Source: CAD feature listing. Evaluate the final solid. Frame: model axes, mm. Face numbers are marked on the shaded views. A direction names the side the tool comes from. Round coordinates to 2 decimals unless told otherwise and drop trailing zeros. Loops run counter-clockwise (first coordinate to the right, second up) from the corner with the lowest first, then second, coordinate; pieces in that order, holes last.
Item 1: Access query for the marked faces 1, 2 and 3. Directions: +Z, -Z, +X, -X, +Y, -Y. A direction counts if a zero-diameter tool reaches every point of the face in a straight line with its end or side. Return the directions, or none.
Item 2: Pull-direction query (Z, two-part tool) for the marked faces 4, 5 and 6; classes: released by +Z, released by -Z, zero draft, split by the parting line, or undercut.
Item 3: Section query A-A on z = 20. Return loops of the section in (x, y), then the cut area to 3 significant figures.
Item 4: Section query B-B on y = 22.5. Return loops of the section in (x, z), then the cut area to 3 significant figures.
Item 5: Section query D-D on y = 15. Return loops of the section in (x, z).
Item 6: Ray query, L1, parallel to X at y = 21.5, z = 8.5; L2, parallel to Y at x = 46.9, z = 80; L3, parallel to Y at x = 40, z = 34.4. Return the intervals inside material, ascending.
Item 7: First-contact query: P1, Ø13, axis at x = 40, y = 65, coming from the +Z side; P2, Ø8, axis at x = 9, z = 14, coming from the +Y side; P3, Ø8, axis at y = 15, z = 80, coming from the -X side; P4, Ø1, axis at x = 41, z = 59.5, coming from the -Y side. Flat tips, straight axial feed; report the tip coordinate or a pass-through.
Item 8: Section query C-C on x = 40. Return loops of the section in (y, z).
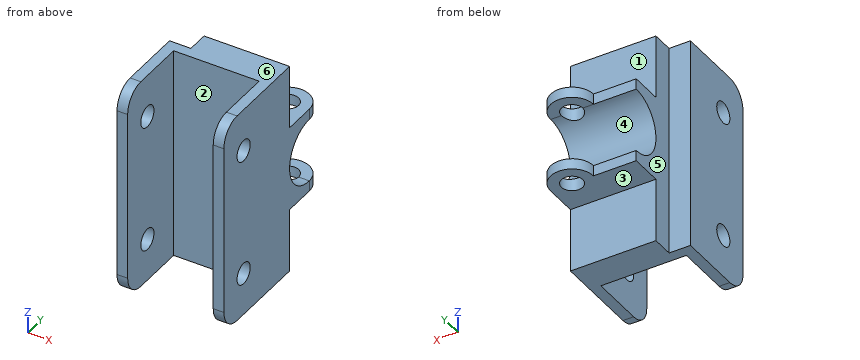
```python
from build123d import *

# Parameters (mm, degrees)
SKETCH1_R               = 5
BOSS_EXTRUDE1_DEPTH     = 100
SKETCH2_R               = 5
SKETCH2_W               = 30
SKETCH2_H               = 25
CUT_EXTRUDE1_DEPTH      = 100
FILLET1_R               = 10
SKETCH4_W               = 40
SKETCH4_H               = 100
BOSS_EXTRUDE2_DEPTH     = 10
SKETCH5_W               = 10
SKETCH5_H               = 20
CUT_EXTRUDE2_DEPTH      = 101
CUT_EXTRUDE2_DEPTH_BACK = 1
SKETCH6_W               = 10
SKETCH6_H               = 5
CUT_EXTRUDE3_DEPTH      = 1
CUT_EXTRUDE3_DEPTH_BACK = 101


with BuildPart() as part:
    # Sketch1 → Boss-Extrude1 (new body)
    with BuildSketch(Plane.XY):
        with BuildLine():
            Line((50, 0), (50, 65))
            ThreePointArc((50, 65), (40, 75), (30, 65))
            Line((30, 65), (0, 65))
            Line((0, 65), (0, 0))
            Line((0, 0), (5, 0))
            Line((5, 0), (5, 45))
            Line((5, 45), (45, 45))
            Line((45, 45), (45, 0))
            Line((45, 0), (50, 0))
        make_face()
        with Locations((40, 65)):
            Circle(SKETCH1_R, mode=Mode.SUBTRACT)
    extrude(amount=BOSS_EXTRUDE1_DEPTH)

    # Sketch2 → Cut-Extrude1 (cut)
    with BuildSketch(Plane(origin=(50, 0, 0), x_dir=(0, 0, -1), z_dir=(1, 0, 0))):
        with Locations((-80, 15)):
            Circle(SKETCH2_R)
        with Locations((-20, 15)):
            Circle(SKETCH2_R)
        with BuildLine():
            Line((-65, 65), (-65, 75))
            Line((-65, 75), (-35, 75))
            Line((-35, 75), (-35, 65))
            ThreePointArc((-35, 65), (-50, 50), (-65, 65))
        make_face()
        with Locations((-85, 62.5)):
            Rectangle(SKETCH2_W, SKETCH2_H)
        with Locations((-15, 62.5)):
            Rectangle(SKETCH2_W, SKETCH2_H)
    extrude(amount=-CUT_EXTRUDE1_DEPTH, mode=Mode.SUBTRACT)

    # Fillet1
    fillet1_edges = [part.edges().sort_by_distance(p)[0] for p in [
        (47.5, 0, 0),
        (2.5, 0, 0),
        (2.5, 0, 100),
        (47.5, 0, 100),
    ]]
    fillet(fillet1_edges, radius=FILLET1_R)

    # Sketch4 → Boss-Extrude2 (add)
    with BuildSketch(Plane.XZ.offset(-45)):
        with Locations((25, 50)):
            Rectangle(SKETCH4_W, SKETCH4_H)
    extrude(amount=BOSS_EXTRUDE2_DEPTH)

    # Sketch5 → Cut-Extrude2 (cut, two sides)
    with BuildSketch(Plane.XY) as cut_extrude2_sk:
        with Locations((5, 55)):
            Rectangle(SKETCH5_W, SKETCH5_H)
    extrude(amount=CUT_EXTRUDE2_DEPTH, mode=Mode.SUBTRACT)
    extrude(cut_extrude2_sk.sketch, amount=-CUT_EXTRUDE2_DEPTH_BACK, mode=Mode.SUBTRACT)

    # Sketch6 → Cut-Extrude3 (cut, two sides)
    with BuildSketch(Plane.XY.offset(100)) as cut_extrude3_sk:
        with Locations((5, 42.5)):
            Rectangle(SKETCH6_W, SKETCH6_H)
    extrude(amount=CUT_EXTRUDE3_DEPTH, mode=Mode.SUBTRACT)
    extrude(cut_extrude3_sk.sketch, amount=-CUT_EXTRUDE3_DEPTH_BACK, mode=Mode.SUBTRACT)


solid = part.part
```
Data:
1. face 1: +Z, +X, -X, +Y
1. face 2: +Z, -Z, -Y
1. face 3: -Z, +X, -X, +Y
2. face 4: undercut
2. face 5: zero draft
2. face 6: released by +Z
3. outline: (0, 0) - (5, 0) - (5, 10) - (0, 10) - close; (0, 20) - (5, 20) - (5, 35) - (45, 35) - (45, 20) - (50, 20) - (50, 50) - (10, 50) - (10, 40) - (0, 40) - close; (45, 0) - (50, 0) - (50, 10) - (45, 10) - close
3. area: 900 mm2
4. outline: (0, 0) - (5, 0) - (5, 100) - (0, 100) - close; (45, 0) - (50, 0) - (50, 100) - (45, 100) - close
4. area: 1,000 mm2
5. outline: (0, 0) - (5, 0) - (5, 15) - (0, 15) - close; (0, 25) - (5, 25) - (5, 75) - (0, 75) - close; (0, 85) - (5, 85) - (5, 100) - (0, 100) - close; (45, 0) - (50, 0) - (50, 15) - (45, 15) - close; (45, 25) - (50, 25) - (50, 75) - (45, 75) - close; (45, 85) - (50, 85) - (50, 100) - (45, 100) - close
6. L1: x = 0 to 5, 45 to 50
6. L2: y = 0 to 10, 20 to 50
6. L3: y = 35 to 60, 70 to 75
7. P1: stops at z = 70
7. P2: stops at y = 50
7. P3: passes through
7. P4: stops at y = 35
8. outline: (35, 0) - (50, 0) - (50, 30) - (60, 30) - (60, 35.86) arc R15 cw to (60, 64.14) - (60, 70) - (50, 70) - (50, 100) - (35, 100) - close; (70, 30) - (75, 30) - (75, 35) - (70, 35) - close; (70, 65) - (75, 65) - (75, 70) - (70, 70) - close
